from build123d import *

# Parameters (mm, degrees)
SKETCH2_R           = 9.5
SKETCH2_R_2         = 2.5
BOSS_EXTRUDE1_DEPTH = 25
SKETCH3_R           = 5
CUT_EXTRUDE1_DEPTH  = 16.5
CUT_EXTRUDE2_DEPTH  = 16.5
SKETCH5_R           = 2
CUT_EXTRUDE3_DEPTH  = 9.5


with BuildPart() as part:
    # Sketch2 → Boss-Extrude1 (new body)
    with BuildSketch(Plane.XY):
        Circle(SKETCH2_R)
        Circle(SKETCH2_R_2, mode=Mode.SUBTRACT)
    extrude(amount=BOSS_EXTRUDE1_DEPTH)

    # Sketch3 → Cut-Extrude1 (cut)
    with BuildSketch(Plane.XY.offset(25)):
        Circle(SKETCH3_R)
    extrude(amount=-CUT_EXTRUDE1_DEPTH, mode=Mode.SUBTRACT)

    # Sketch4 → Cut-Extrude2 (cut)
    with BuildSketch(Plane(origin=(-15.41400196, 54.908076208, -53.970187191), x_dir=(0, 1, 0), z_dir=(1, 0, 0))):
        with BuildLine():
            ThreePointArc((-54.908076208, 58.970187191), (-56.908076208, 56.970187191), (-54.908076208, 54.970187191))
            Line((-54.908076208, 54.970187191), (-54.908076208, 58.970187191))
        make_face()
        with BuildLine():
            Line((-54.908076208, 58.970187191), (-54.908076208, 54.970187191))
            ThreePointArc((-54.908076208, 54.970187191), (-53.493862646, 55.555973629), (-52.908076208, 56.970187191))
            ThreePointArc((-52.908076208, 56.970187191), (-53.493862646, 58.384400753), (-54.908076208, 58.970187191))
        make_face()
        with BuildLine():
            ThreePointArc((-52.908076208, 75.970187191), (-53.493862646, 77.384400753), (-54.908076208, 77.970187191))
            Line((-54.908076208, 77.970187191), (-54.908076208, 73.970187191))
            ThreePointArc((-54.908076208, 73.970187191), (-53.493862646, 74.555973629), (-52.908076208, 75.970187191))
        make_face()
        with BuildLine():
            Line((-54.908076208, 73.970187191), (-54.908076208, 77.970187191))
            ThreePointArc((-54.908076208, 77.970187191), (-56.908076208, 75.970187191), (-54.908076208, 73.970187191))
        make_face()
    extrude(amount=CUT_EXTRUDE2_DEPTH, mode=Mode.SUBTRACT)

    # Sketch5 → Cut-Extrude3 (cut)
    with BuildSketch(Plane(origin=(-15.41400196, -10.091923792, -53.970187191), x_dir=(1, 0, 0), z_dir=(0, -1, 0))):
        with BuildLine():
            ThreePointArc((15.41400196, 58.970187191), (13.41400196, 56.970187191), (15.41400196, 54.970187191))
            Line((15.41400196, 54.970187191), (15.41400196, 58.970187191))
        make_face()
        with BuildLine():
            Line((15.41400196, 58.970187191), (15.41400196, 54.970187191))
            ThreePointArc((15.41400196, 54.970187191), (16.828215523, 55.555973629), (17.41400196, 56.970187191))
            ThreePointArc((17.41400196, 56.970187191), (16.828215523, 58.384400753), (15.41400196, 58.970187191))
        make_face()
        with Locations(Location((15.41400196, 75.970187191, 0), (0, 0, 270))):
            Circle(SKETCH5_R)
    extrude(amount=-CUT_EXTRUDE3_DEPTH, mode=Mode.SUBTRACT)


solid = part.part
Part model, mm, in its own coordinate system. A direction names the side the tool comes from. Coordinates: 2 decimals unless noted, no trailing zeros. Loops run counter-clockwise (first coordinate to the right, second up) from the corner with the lowest first, then second, coordinate; pieces in that order, holes last. Notation, with made-up numbers: (34.5, 1.5) - (55.5, 1.5) arc R14 ccw to (55.5, 27.5) - close; hole circle Ø2 at (-18.5, -19). An arc over 180 degrees is marked (long way). Write each question's results on one line, items separated by ' | '. Start each with the question number.
Q1. Two-plate mould, pull along X, no slides. Class faces 1 (the cylindrical face through (0, -7, 24)), 2 (the flat face through (2, -2, 8.5)), 3 (the cylindrical face through (8.776, -3.639, 12.325)), 4 (the flat face through (2, -2, 0)): +X half, -X half, draft (parallel to the pull), parting line (faces both ways), or undercut.
Q2. Slice it at D-D on y = 4.5. Give the cut face in (x, z), and give its area (3 significant figures).
Q3. Which spindle directions (+Z, -Z, +X, -X, +Y, -Y) get a long thin tool onto all of the face, cutting with end or side? Do faces 5 (the cylindrical face through (4.77, 1.5, 16.87)), 6 (the flat face through (4, -4, 25)). Say none if no direction does.
Q4. Drop flat-ended pins along their axis: pin 1 Ø3 at (y, z) = (2.5, 15.5) entering from +X; pin 2 Ø4 at (x, z) = (7.5, 4) entering from -Y; pin 3 Ø4 at (x, z) = (3.5, 19) entering from -Y; pin 4 Ø3 at (x, y) = (0, 0) entering from +Z. Give the stop position or say it passes through.
Q5. Slice it at C-C on z = 7.5. Give the cut face in (x, y), and give its area (3 significant figures).
Q6. Slice it at B-B on x = -8.5. Give the cut face in (y, z), and give its area (3 significant figures).
Q7. Slice it at A-A on z = 2.5. Give the cut face in (x, y).
Q8. Probe line 1 along Z through (x, y) = (0, -5.7); line 2 along X through (y, z) = (0, 5.25); line 3 along X through (y, z) = (0, 19.5). List the from-to ranges inside material, lowest first.
Answer:
1) face 1: undercut | face 2: undercut | face 3: parting line | face 4: draft
2) outline: (-8.37, 0) - (8.37, 0) - (8.37, 25) - (2.18, 25) - (2.18, 8.5) - (-2.18, 8.5) - (-2.18, 25) - (-8.37, 25) - close | area: 346 mm2
3) face 5: +Z | face 6: +Z, +X, -X, +Y, -Y
4) pin 1: stops at x = 9.45 | pin 2: stops at y = -7.75 | pin 3: stops at y = -9.38 | pin 4: passes through
5) outline: circle Ø19 at (0, 0); hole circle Ø5 at (0, 0) | area: 264 mm2
6) outline: (-4.24, 0) - (4.24, 0) - (4.24, 25) - (-4.24, 25) - close; hole circle Ø4 at (0, 3); hole circle Ø4 at (0, 22) | area: 187 mm2
7) outline: (-9.3, -1.94) arc R9.5 ccw to (-1.94, -9.3) - (-1.94, -1.94) - close; (-9.3, 1.94) - (-1.58, 1.94) arc R2.5 cw to (1.94, -1.58) - (1.94, -9.3) arc R9.5 ccw (long way) to start
8) line 1: z = 0 to 1, 5 to 20, 24 to 25 | line 2: x = -9.5 to -2.5, 2.5 to 9.5 | line 3: x = -9.5 to -5, 5 to 9.5
